Source: CAD feature listing. Evaluate the final solid. Frame: model axes, mm. A direction names the side the tool comes from. Round coordinates to 2 decimals unless told otherwise and drop trailing zeros. Loops run counter-clockwise (first coordinate to the right, second up) from the corner with the lowest first, then second, coordinate; pieces in that order, holes last.
(1) Section A-A, the plane z = 1.2. Return the cut outline in (x, y), plus the area to 3 significant figures.
(2) Material intervals for probe 1 along X at (y, z) = (-7.75, -0.6); probe 2 along X at (y, z) = (-8, -0.3); probe 3 along Y at (x, z) = (4, 0.4), sorted ascending.
(3) Mould query, pull axis X, two halves, no side actions, for faces 6 (the flat face through (6.03, -5.24, -0.74)), 7 (the flat face through (4, -9, 0)), 8 (the flat face through (3.9, 0, 0.8)), 9 (the flat face through (4, -10, 0.5)). Classes: pulls with the +X half, pulls with the -X half, needs draft (parallel to the pull), parting line crosses it, or undercut.
(4) Section C-C, the plane y = -4. Return the cut outline in (x, z), plus the area to 3 significant figures.
(5) First-contact query: pin 1 Ø0.7 at (x, z) = (7.5, 1.5) entering from -Y; pin 2 Ø1.5 at (x, y) = (4, -9) entering from -Z. Flat tips, straight axial feed; report the tip coordinate or a pass-through.
(6) Set-up query: faces 1 (the flat face through (4.98, -9.24, -0.82)), 2 (the flat face through (7.5, -10, 1.5)), 3 (the flat face through (0.9, -5.1, 1.5)), 4 (the flat face through (2.03, -5.1, -0.74)), 5 (the cylindrical face through (5.188, -10.173, 0.493)). Return all of +Z, -Z, +X, -X, +Y, -Y with unobstructed straight access to the full face (end or side cutting, diameter ignored); none if empty.
(7) Section D-D, the plane x = 2.75. Return the cut outline in (y, z).
```python
from build123d import *

# Parameters (mm, degrees)
SKETCH1_W                       = 8
SKETCH1_H                       = 10
BOSS_EXTRUDE1_DEPTH             = 2
SKETCH2_W                       = 6.2
SKETCH2_H                       = 10
CUT_EXTRUDE1_DEPTH              = 1
BOSS_EXTRUDE2_DEPTH             = 1.5
BOSS_EXTRUDE2_DEPTH_BACK        = 1
M1X0_2_TAPPED_HOLE1_D           = 0.8
M1X0_2_TAPPED_HOLE1_DEPTH       = 2.6
M1X0_2_TAPPED_HOLE1_CBORE_D     = 1
M1X0_2_TAPPED_HOLE1_CBORE_DEPTH = 2
M1X0_2_TAPPED_HOLE1_TIP         = 0.240344248
M1_CLEARANCE_HOLE1_D            = 1
M1_CLEARANCE_HOLE1_DEPTH        = 5
M1_CLEARANCE_HOLE1_TIP          = 0.30043031
SKETCH8_R                       = 0.4
CUT_EXTRUDE2_DEPTH              = 1.5
FILLET2_R                       = 1


with BuildPart() as part:
    # Sketch1 → Boss-Extrude1 (new body)
    with BuildSketch(Plane.XY):
        with Locations((4, -5)):
            Rectangle(SKETCH1_W, SKETCH1_H)
    extrude(amount=BOSS_EXTRUDE1_DEPTH)

    # Sketch2 → Cut-Extrude1 (cut)
    with BuildSketch(Plane.XY.offset(2)):
        with Locations((4, -5)):
            Rectangle(SKETCH2_W, SKETCH2_H)
    extrude(amount=-CUT_EXTRUDE1_DEPTH, mode=Mode.SUBTRACT)

    # Sketch3 → Boss-Extrude2 (add, two sides)
    with BuildSketch(Plane(origin=(0, 0, 0), x_dir=(-1, 0, 0), z_dir=(0, 0, -1))) as boss_extrude2_sk:
        Polygon((-8, -10), (-4, -0.343145751), (0, -10), (-2.309698831, -10.956708581), (-4, -6.875960575), (-5.690301169, -10.956708581), align=None)
    extrude(amount=BOSS_EXTRUDE2_DEPTH)
    extrude(boss_extrude2_sk.sketch, amount=-BOSS_EXTRUDE2_DEPTH_BACK)

    # M1x0.2 Tapped Hole1
    with Locations(Plane(origin=(-3.535533906, -8.535533906, 0), x_dir=(-0.923879533, 0.382683432, 0), z_dir=(-0.382683432, -0.923879533, 0))):
        with Locations((-5.115994416, 0.25)):
            CounterBoreHole(M1X0_2_TAPPED_HOLE1_D / 2, M1X0_2_TAPPED_HOLE1_CBORE_D / 2, M1X0_2_TAPPED_HOLE1_CBORE_DEPTH, depth=M1X0_2_TAPPED_HOLE1_DEPTH)
            with Locations((0, 0, -(M1X0_2_TAPPED_HOLE1_DEPTH + M1X0_2_TAPPED_HOLE1_TIP / 2))):  # 118° drill point
                Cone(0, M1X0_2_TAPPED_HOLE1_D / 2, M1X0_2_TAPPED_HOLE1_TIP, mode=Mode.SUBTRACT)

    # M1 Clearance Hole1
    with Locations(Plane(origin=(4.707106781, -11.363961031, 0), x_dir=(-0.923879533, -0.382683432, 0), z_dir=(0.382683432, -0.923879533, 0))):
        with Locations((-2.314201936, 0.25)):
            Hole(M1_CLEARANCE_HOLE1_D / 2, depth=M1_CLEARANCE_HOLE1_DEPTH)
            with Locations((0, 0, -(M1_CLEARANCE_HOLE1_DEPTH + M1_CLEARANCE_HOLE1_TIP / 2))):  # 118° drill point
                Cone(0, M1_CLEARANCE_HOLE1_D / 2, M1_CLEARANCE_HOLE1_TIP, mode=Mode.SUBTRACT)

    # Sketch8 → Cut-Extrude2 (cut)
    with BuildSketch(Plane(origin=(0, 0, -1.5), x_dir=(-1, 0, 0), z_dir=(0, 0, -1))):
        with Locations((-4, -7.3)):
            Circle(SKETCH8_R)
    extrude(amount=-CUT_EXTRUDE2_DEPTH, mode=Mode.SUBTRACT)

    # Fillet2
    fillet2_edges = [part.edges().sort_by_distance(p)[0] for p in [
        (2.705980501, -10, 0.5),
        (5.294019499, -10, 0.5),
    ]]
    fillet(fillet2_edges, radius=FILLET2_R)


solid = part.part
```
Output values:
1. outline: (0, -10) - (0.9, -10) - (0.9, 0) - (0, 0) - close; (7.1, -10) - (8, -10) - (8, 0) - (7.1, 0) - close
1. area: 18.0 mm2
2. probe 1: x = 0.93 to 3.64, 4.36 to 5.33, 6.1 to 7.07
2. probe 2: x = 0.83 to 1.79, 2.37 to 3.53, 4.47 to 5.28, 6.36 to 7.17
2. probe 3: y = -10 to 0
3. face 6: pulls with the +X half
3. face 7: undercut
3. face 8: needs draft
3. face 9: undercut
4. outline: (0, 0) - (2.49, 0) - (2.49, -1.5) - (5.51, -1.5) - (5.51, 0) - (8, 0) - (8, 2) - (7.1, 2) - (7.1, 1) - (0.9, 1) - (0.9, 2) - (0, 2) - close
4. area: 14.3 mm2
5. pin 1: stops at y = -10
5. pin 2: stops at z = 0
6. face 1: -Z, -Y
6. face 2: +Z, +X, -X, -Y
6. face 3: +Z, +Y, -Y
6. face 4: -Z, -X, +Y
6. face 5: +Z, -Z, -Y
7. outline: (-10.22, 0) - (-9.89, 0) - (-9.89, -1.5) - (-3.36, -1.5) - (-3.36, 0) - (0, 0) - (0, 1) - (-10.22, 1) - close
